The figure shows three views and two pictorial views of one solid part (mm, origin at its lowest corner). Answer the questions. Round coordinates to 2 decimals unless told otherwise and drop trailing zeros. Write each loop counter-clockwise with the first axis right and the second up, starting at its lowest first coordinate (ties: lowest second). Pieces come first, ordered by that corner, then holes. Notation, with made-up numbers: M 0,15 L 12,15 A29 cw 12,52 Z; hole C 47,38 d10. An arc over 180 degrees is marked long. One line per item, written item: value. Start each with the question number.
Q1. Find section A-A (y = 82.5). Write down the section's boundary in (x, z), and give its area (3 significant figures).
Q2. Find section B-B (x = 60). Write down the section's boundary in (y, z).
Q3. Consider probe 1 along Y at (x, z) = (60, 1.2); probe 2 along Y at (x, z) = (10, 2.25); probe 3 along X at (y, z) = (82.5, 2.05). Determine where each line is inside the solid, lowest interval first.
Q4. Given pin 1 Ø5 at (x, y) = (60, 90) entering from +Z, flat-ended and moving along its own axis, determine where the tip first touches the part or whether it passes through.
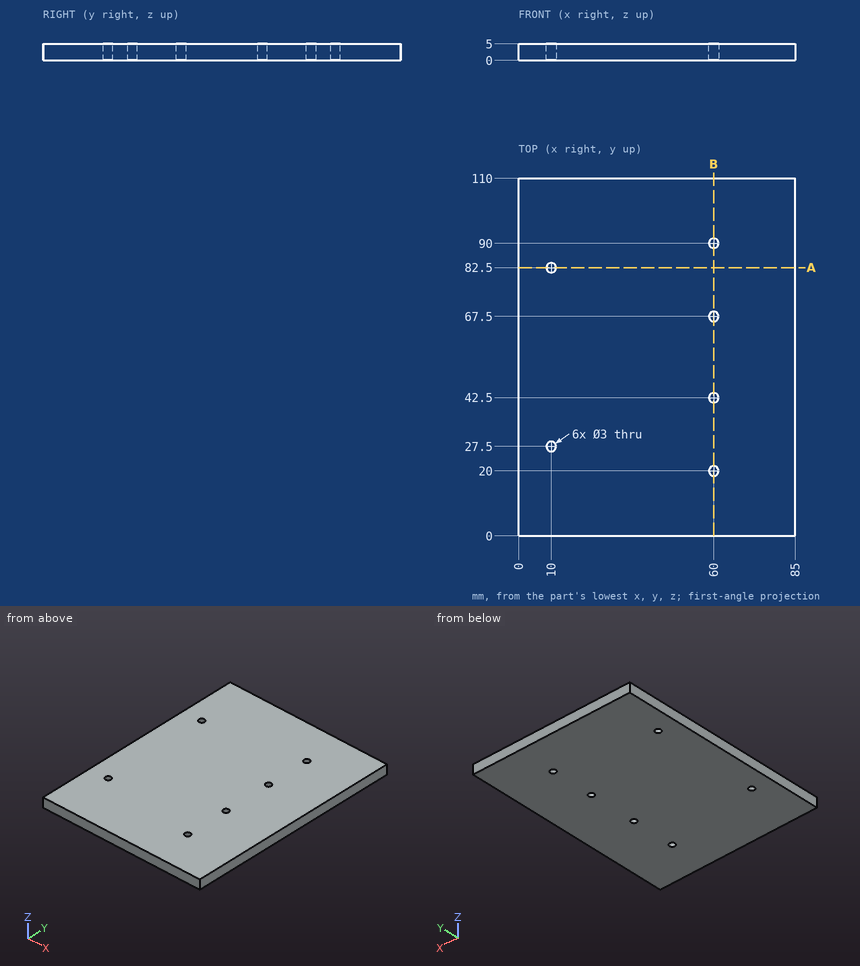
The answers:
1. outline: M 0,0 L 8.5,0 L 8.5,5 L 0,5 Z; M 11.5,0 L 85,0 L 85,5 L 11.5,5 Z
1. area: 410 mm2
2. outline: M 0,0 L 18.5,0 L 18.5,5 L 0,5 Z; M 21.5,0 L 41,0 L 41,5 L 21.5,5 Z; M 44,0 L 66,0 L 66,5 L 44,5 Z; M 69,0 L 88.5,0 L 88.5,5 L 69,5 Z; M 91.5,0 L 110,0 L 110,5 L 91.5,5 Z
3. probe 1: 0 to 18.5, 21.5 to 41, 44 to 66, 69 to 88.5, 91.5 to 110
3. probe 2: 0 to 26, 29 to 81, 84 to 110
3. probe 3: 0 to 8.5, 11.5 to 85
4. pin 1: z = 5
